Autodesk Inventor part; units mm, degrees
ref_plane "Work Plane1" through (130.8625, -3.3799, 0) normal (0, 0, 1) x (1, 0, 0)
ref_plane "YZ Plane" through (0, 0, 0) normal (1, 0, 0) x (0, 1, 0)
ref_plane "XZ Plane" through (0, 0, 0) normal (0, 1, 0) x (-1, 0, 0)
sketch "Sketch1" plane through (0, 0, 0) normal (0, 0, 1) x (1, 0, 0)
  line L0 (-23.9187, 7.7326) -> (57.0438, 7.7326)
  line L1 (63.3938, 7.7326) -> (63.3938, 18.8451)
  line L2 (63.3938, 18.8451) -> (72.9188, 18.8451)
  line L3 (72.9188, 18.8451) -> (72.9188, 7.7326)
  line L4 (72.9188, 7.7326) -> (112.6063, 7.7326)
  line L5 (112.6063, 7.7326) -> (112.6063, 18.8451)
  line L6 (112.6063, 18.8451) -> (149.1188, 18.8451)
  line L7 (149.1188, 18.8451) -> (149.1188, -3.3799)
  line L8 (149.1188, -3.3799) -> (-23.9187, -3.3799)
  line L9 (-23.9187, -3.3799) -> (-23.9187, 7.7326)
  line L10 (57.0438, 7.7326) -> (57.0438, 6.1451)
  line L11 (57.0438, 6.1451) -> (63.3938, 6.1451)
  line L12 (63.3938, 6.1451) -> (63.3938, 7.7326)
  dimension "d0" = 11.1125
  dimension "d1" = 22.225
  dimension "d2" = 11.1125
  dimension "d3" = 9.525
  dimension "d4" = 173.0375
  dimension "d5" = 36.5125
  dimension "d6" = 39.6875
  dimension "d7" = 6.35
  dimension "d8" = 9.525
revolve "Revolution1" add sketch "Sketch1" angle 360 about axis through (149.1188, -3.3799, 0) along (-1, 0, 0)
chamfer "Chamfer1" distance 1.5875 angle 45 1 edges at (-23.9187, -14.4924, 0)
sketch "Sketch2" plane through (149.1188, -3.3799, 0) normal (1, 0, 0) x (0, 0, -1)
  circle A0 centre (0, 0) radius 22.225
  line L0 (14.4087, 21.2365) -> (25.5957, -1.8601)
  line L1 (25.5957, -1.8601) -> (11.187, -23.0966)
  line L2 (11.187, -23.0966) -> (-14.4087, -21.2365)
  line L3 (-14.4087, -21.2365) -> (-25.5957, 1.8601)
  line L4 (-25.5957, 1.8601) -> (-11.187, 23.0966)
  line L5 (-11.187, 23.0966) -> (14.4087, 21.2365)
  dimension "d12" = 44.45
extrude "Extrusion1" add sketch "Sketch2" against normal blind 12.7 contours A0 L0 L1 | A0 L5 L0 | L1 L2 A0 | A0 L4 L5 | L2 L3 A0 | A0 L3 L4
ref_plane "Work Plane1" through (130.8625, -3.3799, 0) normal (0, 0, 1) x (1, 0, 0)
sketch "Sketch3" plane through (130.8625, -3.3799, 0) normal (0, 0, 1) x (1, 0, 0)
  line L0 (18.2563, 23.0966) -> (5.5563, 23.0966)
  line L1 (18.2563, 1.8601) -> (18.2563, 23.0966)
  line L2 (12.9718, 32.2495) -> (24.7507, 11.8479)
  line L3 (12.9718, 32.2495) -> (24.7507, 32.2495)
  line L4 (24.7507, 32.2495) -> (24.7507, 11.8479)
  line L5 (-172.7344, 0) -> (78.6103, 0)
  dimension "d16" = 30
revolve "Revolution2" cut sketch "Sketch3" angle 360 about axis through (130.8625, -3.3799, 0) along (1, 0, 0)
thread "Thread1"
properties part number "Wedge_Screw"
Can you work these out from the model? Positions are in its coordinate system, mm. A direction names the side the tool comes from. Round coordinates to 2 decimals unless told otherwise and drop trailing zeros. Order: outer loops, then holes, each group sorted by start corner. A loop starts at its lowest first (then second) coordinate and runs counter-clockwise, first axis right, second up. Notation, with made-up numbers: (52, 12) -> (71, 12) arc R22 ccw to (71, 33) -> close; hole circle Ø1 at (60.25, 59.5). An arc over 180 degrees is marked (long way). Write each question's results on one line, items separated by ' | '. Start each with the question number.
Item 1: Thinking about a two-plate mould opening in X: for faces 1 (the cylindrical face through (60.263, 5.705, 2.861)), 2 (the flat face through (136.419, 17, 10)), 3 (the flat face through (142.86, 8.95, 18.49)), which applies, +X half, -X half, draft (parallel to the pull), parting line (faces both ways), or undercut?
Item 2: Will these pins go through, and if not, where does the flat tip stop? pin 1 (1 mm diameter, centred on x = 76, y = -7.5, fed in from +Z); pin 2 (10 mm diameter, centred on x = 67.5, y = 7, fed in from -Z); pin 3 (3.5 mm diameter, centred on y = 10.5, z = -11.5, fed in from -X).
Item 3: If we section it at A-A, the plane z = 0: Write out the boundary of the cut face in (x, y), then the cut area to 3 significant figures.
Item 4: If we section it at B-B, the plane x = 96: Write out the boundary of the cut face in (y, z) (1 decimal).
Item 5: Please list where these lines run through material, in increasing order: L1, parallel to X at y = 4, z = 13; L2, parallel to Y at x = 19, z = 5.5; L3, parallel to Z at x = 0.5, y = -3.
Item 6: Which directions (+Z, -Z, +X, -X, +Y, -Y) give clear straight access to the entire face, cutting with the end or side of a thin tool? Please do faces 4 (the flat face through (72.919, -14, 5)), 5 (the cylindrical face through (17.91, -14.48, 0.49)), 6 (the conical face through (148.7, 16.38, -13.31)).
Results:
1) face 1: undercut | face 2: -X half | face 3: draft
2) pin 1: stops at z = 10.51 | pin 2: stops at z = -21.56 | pin 3: stops at x = 63.39
3) outline: (-23.92, -12.9) -> (-22.33, -14.49) -> (57.04, -14.49) -> (57.04, -12.9) -> (63.39, -12.9) -> (63.39, -25.6) -> (72.92, -25.6) -> (72.92, -14.49) -> (112.61, -14.49) -> (112.61, -25.6) -> (136.42, -25.6) -> (136.42, -25.66) -> (149.12, -25.66) -> (149.12, 18.9) -> (136.42, 18.9) -> (136.42, 18.85) -> (112.61, 18.85) -> (112.61, 7.73) -> (72.92, 7.73) -> (72.92, 18.85) -> (63.39, 18.85) -> (63.39, 6.15) -> (57.04, 6.15) -> (57.04, 7.73) -> (-22.33, 7.73) -> (-23.92, 6.15) -> close | area: 4,850 mm2
4) outline: circle Ø22.2 at (-3.4, 0)
5) L1: x = 63.39 to 72.92, 112.61 to 149.12 | L2: y = -13.04 to 6.28 | L3: z = -11.11 to 11.11
6) face 4: none | face 5: -X | face 6: -Z, +X, +Y
